The model under review builds one solid part; all positions refer to its coordinate system, in mm. Face numbers are marked on the shaded views. A direction names the side the tool comes from. Round coordinates to 2 decimals unless told otherwise and drop trailing zeros. Order: outer loops, then holes, each group sorted by start corner. A loop starts at its lowest first (then second) coordinate and runs counter-clockwise, first axis right, second up. Notation, with made-up numbers: M -4,41 L 8,41 A14 ccw 8,60 Z; hole C 84,62.25 d4. An arc over 180 degrees is marked long. Answer as a JSON object with one key per item and string values. Group by question number.
1. Clearance check with flat-ended pins moving along their axes: P1, Ø1.3, axis at y = 5, z = -14, coming from the -X side; P2, Ø12, axis at x = 23.5, y = -10, coming from the +Z side (3 decimals); P3, Ø7.5, axis at x = -22, y = 0, coming from the +Z side (3 decimals). State where each tip first meets the part, or that it passes through.
2. Mouldability with a two-part tool opening along X and no side actions: class the marked faces 3, 4, 5 and 6 as released by +X, released by -X, zero draft, split by the parting line, or undercut.
3. To check wall thickness, follow probe 1 along X at (y, z) = (-13, 7); probe 2 along Y at (x, z) = (23, 3) (3 decimals); probe 3 along Y at (x, z) = (-18, 3) (3 decimals). State the ranges of each line that lie inside material, in increasing order. Write a range as [from, to].
4. Add section A-A on z = 4. Give the number of separate pieces and of enclosed holes in the cut face, and give its area (3 significant figures).
5. Add section B-B on x = -36. State the section outline as (y, z) points (3 decimals).
6. Machinability: for the marked faces 1 and 2, which of the approach directions +Z, -Z, +X, -X, +Y, -Y give a long, thin tool a straight path to every point of the face, cutting with its end or side? Answer none if there is none.
7. Add section C-C on x = 65.5. State the section outline as (y, z) points (3 decimals).
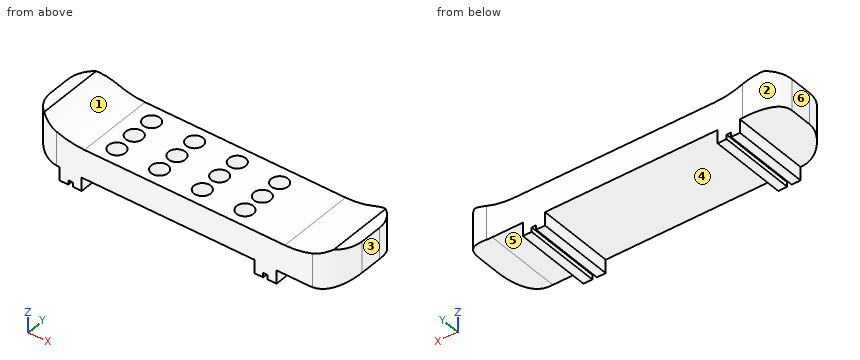
```python
from build123d import *

# Parameters (mm, degrees)
F0_W          = 177.8
F0_H          = 31.75
F12_DEPTH     = 22.225
F1_W          = 2.54
F1_H          = 2.54
F2_DEPTH      = 22.225
F2_DEPTH_BACK = 22.225
F3_W          = 17.4625
F3_H          = 7.62
F3_W_2        = 98.425
F3_W_3        = 36.5125
F4_DEPTH      = 44.451
F6_DEPTH      = 44.451
F7_R          = 15.875
F9_D          = 9.525
F10_W         = 98.425
F10_H         = 44.45
F11_DEPTH     = 2.54


# Not quite as in the source:
# - a length typed as a fraction of an inch, garbled in the dataset ("3 / 203.2 mm" for 3/8 in), is restored


with BuildPart() as f12:
    # F0 (on Front) → F12 (new body, symmetric)
    with BuildSketch(Plane.XZ):
        Rectangle(F0_W, F0_H)
    extrude(amount=F12_DEPTH, both=True)

    # F1 (on Front) → F2 (cut, two sides)
    with BuildSketch(Plane.XZ) as f2_sk:
        with Locations((-65.0875, -14.605)):
            Rectangle(F1_W, F1_H)
        with Locations((46.0375, -14.605)):
            Rectangle(F1_W, F1_H)
    extrude(amount=F2_DEPTH, mode=Mode.SUBTRACT)
    extrude(f2_sk.sketch, amount=-F2_DEPTH_BACK, mode=Mode.SUBTRACT)

    # F3 (on face) → F4 (cut, through all)
    with BuildSketch(Plane.XZ.offset(22.225)):
        with Locations((-80.16875, -12.065)):
            Rectangle(F3_W, F3_H)
        with Locations((-9.525, -12.065)):
            Rectangle(F3_W_2, F3_H)
        with Locations((70.64375, -12.065)):
            Rectangle(F3_W_3, F3_H)
    extrude(amount=-F4_DEPTH, mode=Mode.SUBTRACT)

    # F5 (on face) → F6 (cut, through all)
    with BuildSketch(Plane.XZ.offset(22.225)):
        with BuildLine():
            Line((82.55, 15.875), (-82.55, 15.875))
            ThreePointArc((-82.55, 15.875), (-70.4091892663, 10.2010357789), (-57.15, 8.255))
            Line((-57.15, 8.255), (57.15, 8.255))
            ThreePointArc((57.15, 8.255), (70.4091892663, 10.2010357789), (82.55, 15.875))
        make_face()
        with BuildLine():
            ThreePointArc((-71.12, -8.255), (-80.5599536545, -6.6198702327), (-88.9, -1.905))
            Line((-88.9, -1.905), (-88.9, -8.255))
            Line((-88.9, -8.255), (-71.4375, -8.255))
            Line((-71.4375, -8.255), (-71.12, -8.255))
        make_face()
        with BuildLine():
            Line((88.9, -8.255), (88.9, -1.905))
            ThreePointArc((88.9, -1.905), (79.890231571, -6.6256947131), (69.85, -8.255))
            Line((69.85, -8.255), (88.9, -8.255))
        make_face()
    extrude(amount=-F6_DEPTH, mode=Mode.SUBTRACT)

    # F7
    f7_edges = [f12.edges().sort_by_distance(p)[0] for p in [
        (-88.9, -22.225, 6.985),
        (88.9, -22.225, 6.985),
        (88.9, 22.225, 6.985),
        (-88.9, 22.225, 6.985),
    ]]
    fillet(f7_edges, radius=F7_R)

    # F9 (through all)
    with Locations(Plane(origin=(0, 0, -8.255), x_dir=(1, 0, 0), z_dir=(0, 0, -1))):
        with Locations((-46.0375, 12.7), (-46.0375, 0), (-46.0375, -12.7), (26.9875, -12.7), (26.9875, 0), (26.9875, 12.7), (-21.6958333333, 12.7), (2.6458333333, 12.7), (2.6458333333, 0), (-21.6958333333, 0), (-21.6958333333, -12.924679948), (2.6458333333, -12.924679948)):
            Hole(F9_D / 2)

    # F10 (on face) → F11 (join)
    with BuildSketch(Plane(origin=(0, 0, -8.255), x_dir=(1, 0, 0), z_dir=(0, 0, -1))):
        with Locations((-9.525, 0)):
            Rectangle(F10_W, F10_H)
    extrude(amount=-F11_DEPTH)


solid = f12.part
```
Recorded:
{
 "1": {"P1": "stops at x = -71.44", "P2": "stops at z = 8.255", "P3": "stops at z = -5.715"},
 "2": {"face 3": "released by +X", "face 4": "undercut", "face 5": "zero draft", "face 6": "released by -X"},
 "3": {"probe 1": "x = [-87.44, -50.79], [-41.28, -26.45], [-16.94, -2.11], [7.4, 22.23], [31.74, 87.44]", "probe 2": "y = [-22.225, -15.304], [-10.096, -2.604], [2.604, 10.096], [15.304, 22.225]", "probe 3": "y = [-22.225, -15.704], [-9.696, -3.004], [3.004, 9.921], [15.928, 22.225]"},
 "4": {"separate pieces": "1", "enclosed holes": "12", "area": "6,830 mm²"},
 "5": {"outline": "M -22.225,-8.255 L 22.225,-8.255 L 22.225,8.255 L -22.225,8.255 Z"},
 "6": {"face 1": "+Z, +Y, -Y", "face 2": "+Z, -Z, -X, +Y"},
 "7": {"outline": "M -22.225,-8.255 L 22.225,-8.255 L 22.225,9.017 L -22.225,9.017 Z"}
}
